Check sheet for the modelled part. Datum: model origin and axes. Units: mm. Face numbers are marked on the shaded views. A direction names the side the tool comes from. Round coordinates to 2 decimals unless told otherwise and drop trailing zeros. Write each loop counter-clockwise with the first axis right and the second up, starting at its lowest first coordinate (ties: lowest second). Pieces come first, ordered by that corner, then holes. Notation, with made-up numbers: M 47.5,46.25 L 79.5,46.25 A29 ccw 79.5,68.25 Z; hole C -11,22 d9. An arc over 180 degrees is marked long. Answer in a Markdown table with one row per item.
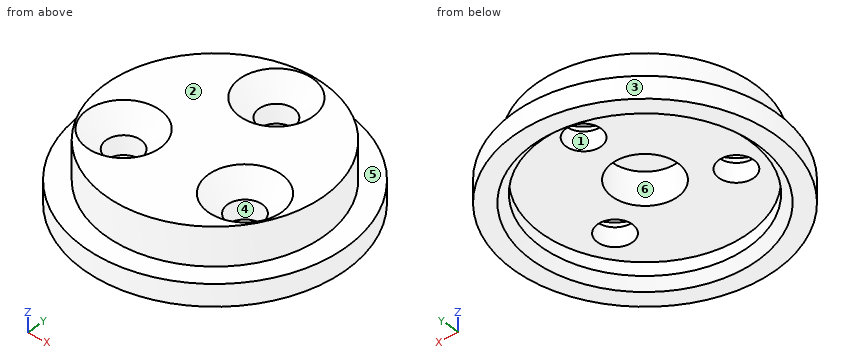
```python
from build123d import *

# Parameters (mm, degrees)
CSK_FOR_M3_SFHCS1_D           = 3.2
CSK_FOR_M3_SFHCS1_CSINK_D     = 6.72
CSK_FOR_M3_SFHCS1_CSINK_ANGLE = 90
CHAMFER1_SIZE                 = 0.8


with BuildPart() as part:
    # Sketch1 → Revolve1 (revolve)
    with BuildSketch(Plane(origin=(0, 0, 0), x_dir=(1, 0, 0), z_dir=(0, 1, 0))):
        Polygon((0, 0), (3, 0), (3, 3), (9.5, 3), (9.5, 5), (12, 5), (12, 3), (10, 3), (10, -0.5), (0, -0.5), align=None)
    revolve(axis=Axis((0, 0, 0), (0, 0, -1)))

    # CSK for M3 SFHCS1 (through all)
    with Locations(Plane.XY.offset(0.5)):
        with Locations((0, 6.5), (5.629165125, -3.25), (-5.629165125, -3.25)):
            CounterSinkHole(CSK_FOR_M3_SFHCS1_D / 2, CSK_FOR_M3_SFHCS1_CSINK_D / 2, counter_sink_angle=CSK_FOR_M3_SFHCS1_CSINK_ANGLE)

    # Chamfer1
    chamfer1_edges = [part.edges().sort_by_distance(p)[0] for p in [
        (-9.5, 0, -5),
    ]]
    chamfer(chamfer1_edges, length=CHAMFER1_SIZE)


solid = part.part
```
1. Section check D-D, the plane z = -0.65. Record the cut outline in (x, y).
Found:
| item | result |
|---|---|
| outline | C 0,0 d20; hole C -5.63,-3.25 d4.42; hole C 0,0 d6; hole C 0,6.5 d4.42; hole C 5.63,-3.25 d4.42 |
2. Scan lines: L1, parallel to Y at x = 0, z = -1.9; L2, parallel to Y at x = 0, z = -3.5; L3, parallel to X at y = -4.5, z = -2. Record each from-to range of solid material in increasing order.
Found:
| item | result |
|---|---|
| L1 | y = -10 to -3, 3 to 4.9, 8.1 to 10 |
| L2 | y = -12 to -9.5, 9.5 to 12 |
| L3 | x = -8.93 to -6.63, -4.63 to 4.63, 6.63 to 8.93 |
3. Section check C-C, the plane z = -3.5. Record the cut outline in (x, y).
Found:
| item | result |
|---|---|
| outline | C 0,0 d24; hole C 0,0 d19 |
4. Access from +Z, -Z, +X, -X, +Y, -Y to the whole of each face (thin tool, end or side, straight path). Record for the marked faces 4, 5 and 6.
Found:
| item | result |
|---|---|
| face 4 | +Z, -Z |
| face 5 | +Z |
| face 6 | -Z |
5. Draft check along Y on the marked faces 1, 2 and 3. Enter one of: +Y half, -Y half, draft (parallel to the pull), parting line (faces both ways), or undercut.
Found:
| item | result |
|---|---|
| face 1 | undercut |
| face 2 | draft |
| face 3 | parting line |
6. Go/stop test with flat-tipped pins: pin 1 (3 mm diameter, centred on x = -0.5, y = 0.5, fed in from -Z); pin 2 (4 mm diameter, centred on x = 0, y = 6.5, fed in from -Z). Record where each tip stops, or that it passes through.
Found:
| item | result |
|---|---|
| pin 1 | stops at z = 0 |
| pin 2 | stops at z = -3 |
7. Section check B-B, the plane z = -2.15. Record the cut outline in (x, y).
Found:
| item | result |
|---|---|
| outline | C 0,0 d20; hole C -5.63,-3.25 d3.2; hole C 0,0 d6; hole C 0,6.5 d3.2; hole C 5.63,-3.25 d3.2 |
8. Section check A-A, the plane x = 0. Record the cut outline in (y, z), and give its area (3 significant figures).
Found:
| item | result |
|---|---|
| outline | M -12,-5 L -10.3,-5 L -9.5,-4.2 L -9.5,-3 L -3,-3 L -3,0 L 3,0 L 3,-3 L 4.9,-3 L 4.9,-1.26 L 3.14,0.5 L -10,0.5 L -10,-3 L -12,-3 Z; M 8.1,-3 L 9.5,-3 L 9.5,-4.2 L 10.3,-5 L 12,-5 L 12,-3 L 10,-3 L 10,0.5 L 9.86,0.5 L 8.1,-1.26 Z |
| area | 47.1 mm2 |
